from build123d import *

# Parameters (mm, degrees)
SKETCH1_W           = 63.5
SKETCH1_H           = 35
SKETCH1_R           = 1.13
SKETCH1_W_2         = 8.85
SKETCH1_H_2         = 31.2
SKETCH1_R_2         = 2.144603346
BOSS_EXTRUDE1_DEPTH = 0.508


with BuildPart() as part:
    # Sketch1 → Boss-Extrude1 (new body)
    with BuildSketch(Plane(origin=(0, 0, 0), x_dir=(1, 0, 0), z_dir=(0, 1, 0))):
        Rectangle(SKETCH1_W, SKETCH1_H)
        with BuildLine():
            Line((-2.5, 5.075), (-2.5, 12.075))
            Line((-2.5, 12.075), (2.5, 12.075))
            Line((2.5, 12.075), (2.5, 5.075))
            Line((2.5, 5.075), (7.575, 5.075))
            ThreePointArc((7.575, 5.075), (6.842766953, 3.307233047), (5.075, 2.575))
            Line((5.075, 2.575), (5.075, -2.575))
            ThreePointArc((5.075, -2.575), (6.842766953, -3.307233047), (7.575, -5.075))
            Line((7.575, -5.075), (2.5, -5.075))
            Line((2.5, -5.075), (2.5, -12.075))
            Line((2.5, -12.075), (-2.5, -12.075))
            Line((-2.5, -12.075), (-2.5, -5.075))
            Line((-2.5, -5.075), (-7.575, -5.075))
            ThreePointArc((-7.575, -5.075), (-6.842766953, -3.307233047), (-5.075, -2.575))
            Line((-5.075, -2.575), (-5.075, 2.575))
            ThreePointArc((-5.075, 2.575), (-6.842766953, 3.307233047), (-7.575, 5.075))
            Line((-7.575, 5.075), (-2.5, 5.075))
        make_face(mode=Mode.SUBTRACT)
        with Locations(Location((-18, -8.5, 0), (0, 0, 270))):
            Circle(SKETCH1_R, mode=Mode.SUBTRACT)
        with Locations(Location((18, -8.5, 0), (0, 0, 270))):
            Circle(SKETCH1_R, mode=Mode.SUBTRACT)
        with Locations((-24.825, 0)):
            Rectangle(SKETCH1_W_2, SKETCH1_H_2, mode=Mode.SUBTRACT)
        with Locations(Location((-18.034, 0, 0), (0, 0, 270))):
            Circle(SKETCH1_R_2, mode=Mode.SUBTRACT)
        with Locations(Location((-18, 8.5, 0), (0, 0, 270))):
            Circle(SKETCH1_R, mode=Mode.SUBTRACT)
        with Locations(Location((18, 8.5, 0), (0, 0, 270))):
            Circle(SKETCH1_R, mode=Mode.SUBTRACT)
        with Locations((24.825, 0)):
            Rectangle(SKETCH1_W_2, SKETCH1_H_2, mode=Mode.SUBTRACT)
        with Locations(Location((18.034, 0, 0), (0, 0, 270))):
            Circle(SKETCH1_R_2, mode=Mode.SUBTRACT)
    extrude(amount=BOSS_EXTRUDE1_DEPTH)


solid = part.part
Geometry check sheet. Reference: the model listing, model coordinates, mm. A direction names the side the tool comes from. Give positions to 0.01 mm unless a question says otherwise; leave off trailing zeros. Write each loop counter-clockwise with the first axis right and the second up, starting at its lowest first coordinate (ties: lowest second). Pieces come first, ordered by that corner, then holes. Notation, with made-up numbers: M 31.25,-10.5 L 87.25,-10.5 A27 ccw 87.25,28.5 Z; hole C 32.5,-1 d4. An arc over 180 degrees is marked long. Answer as CSV lines item,"result". Start each with the question number.
Q1. Section check C-C, the plane z = 11. Record the cut outline in (x, y), then the cut area to 3 significant figures.
Q2. Section check B-B, the plane x = -21. Record the cut outline in (y, z), then the cut area to 3 significant figures.
Q3. Section check D-D, the plane y = 0.3. Give the number of separate pieces and of enclosed holes in the cut face, then the cut area to 3 significant figures.
Q4. Tool access check on faces 1 (the face through (-8, 0.508, 0)), 2 (the face through (6.862, 0.25, -3.327)). Record the directions out of +Z, -Z, +X, -X, +Y, -Y that give a thin tool (end or side, any length) a straight path to the whole face; none if there is none.
Q5. Material ranges on L1, parallel to X at y = 0.45, z = 8.5; L2, parallel to X at y = 0.4, z = 0 (3 decimals); L3, parallel to X at y = 0.2, z = -15.5, recorded low to high.
Q6. Release check for a two-part mould opening along Z. For faces 3 (the face through (-18.433, 0.25, -7.456)), 4 (the face through (-8, 0, 0)) record: pulls with the +Z half, pulls with the -Z half, needs draft (parallel to the pull), parting line crosses it, or undercut.
Q7. Section check A-A, the plane z = -8.5. Record the cut outline in (x, y), then the cut area to 3 significant figures.
Geometry says:
1,outline,"M -31.75,0 L -29.25,0 L -29.25,0.51 L -31.75,0.51 Z; M -20.4,0 L -2.5,0 L -2.5,0.51 L -20.4,0.51 Z; M 2.5,0 L 20.4,0 L 20.4,0.51 L 2.5,0.51 Z; M 29.25,0 L 31.75,0 L 31.75,0.51 L 29.25,0.51 Z"
1,area,"20.7 mm^2"
2,outline,"M 0,-17.5 L 0.51,-17.5 L 0.51,-15.6 L 0,-15.6 Z; M 0,15.6 L 0.51,15.6 L 0.51,17.5 L 0,17.5 Z"
2,area,"1.93 mm^2"
3,separate pieces,"1"
3,enclosed holes,"9"
3,area,"1,430 mm^2"
4,face 1,"+Z, -Z, +X, -X, +Y"
4,face 2,"+Y, -Y"
5,L1,"-31.75 to -29.25, -20.4 to -19.13, -16.87 to -2.5, 2.5 to 16.87, 19.13 to 20.4, 29.25 to 31.75"
5,L2,"-31.75 to -29.25, -20.4 to -20.179, -15.889 to -5.075, 5.075 to 15.889, 20.179 to 20.4, 29.25 to 31.75"
5,L3,"-31.75 to -29.25, -20.4 to 20.4, 29.25 to 31.75"
6,face 3,"undercut"
6,face 4,"needs draft"
7,outline,"M -31.75,0 L -29.25,0 L -29.25,0.51 L -31.75,0.51 Z; M -20.4,0 L -19.13,0 L -19.13,0.51 L -20.4,0.51 Z; M -16.87,0 L -2.5,0 L -2.5,0.51 L -16.87,0.51 Z; M 2.5,0 L 16.87,0 L 16.87,0.51 L 2.5,0.51 Z; M 19.13,0 L 20.4,0 L 20.4,0.51 L 19.13,0.51 Z; M 29.25,0 L 31.75,0 L 31.75,0.51 L 29.25,0.51 Z"
7,area,"18.4 mm^2"
